```python
from build123d import *

# Parameters (mm, degrees)
BOSS_EXTRUDE1_DEPTH = 5.9944
CHAMFER1_SIZE       = 3.175


with BuildPart() as part:
    # Sketch1 → Boss-Extrude1 (new body)
    with BuildSketch(Plane(origin=(0, 0, 0), x_dir=(1, 0, 0), z_dir=(0, 1, 0))):
        Polygon((-53.975, 0), (-6.35, 0), (-6.35, -3.175), (-3.175, -3.175), (-3.175, 0), (0, 0), (0, 12.7), (-3.175, 12.7), (-3.175, 15.875), (-6.35, 15.875), (-6.35, 12.7), (-53.975, 12.7), (-53.975, 15.875), (-57.15, 15.875), (-57.15, 19.05), (-69.85, 19.05), (-69.85, 15.875), (-73.025, 15.875), (-73.025, 12.7), (-120.65, 12.7), (-120.65, 15.875), (-123.825, 15.875), (-123.825, 12.7), (-127, 12.7), (-127, 0), (-123.825, 0), (-123.825, -3.175), (-120.65, -3.175), (-120.65, 0), (-73.025, 0), (-73.025, -3.175), (-69.85, -3.175), (-69.85, -6.35), (-57.15, -6.35), (-57.15, -3.175), (-53.975, -3.175), align=None)
    extrude(amount=BOSS_EXTRUDE1_DEPTH)

    # Chamfer1
    chamfer1_edges = [part.edges().sort_by_distance(p)[0] for p in [
        (-6.35, 2.9972, -12.7),
        (-6.35, 2.9972, 0),
        (-120.65, 2.9972, 0),
        (-120.65, 2.9972, -12.7),
    ]]
    chamfer(chamfer1_edges, length=CHAMFER1_SIZE - 0.0001)  # a hair under: the kernel refuses the full size


solid = part.part
```
Read the model definition and answer for the solid it produces. Units are mm, in the model's axes. A direction names the side the tool comes from. Give positions to 0.01 mm unless a question says otherwise; leave off trailing zeros. Order: outer loops, then holes, each group sorted by start corner. A loop starts at its lowest first (then second) coordinate and runs counter-clockwise, first axis right, second up.
(1) For a pull along X with two mould halves and no side action, classify faces 4 (the flat face through (-96, 3, 0)), 5 (the flat face through (-56, 3, 3.175)), 6 (the flat face through (-123.825, 3, -14)), 7 (the flat face through (-3.175, 3, 2)) as released by +X, released by -X, zero draft, split by the parting line, or undercut.
(2) Given pin 1 (3 mm diameter, centred on x = -30, y = 2.5, fed in from +Z); pin 2 (2.5 mm diameter, centred on y = 2, z = 4, fed in from -X) (3 decimals); pin 3 (3 mm diameter, centred on x = -23.5, y = 2, fed in from -Z); pin 4 (10 mm diameter, centred on x = -44.5, z = -3.5, fed in from -Y), each flat-ended and moving along its own axis, determine where each tip first touches the part or whether it passes through.
(3) Straight lines are drawn through the part: L1, parallel to X at y = 3.3, z = 1 (3 decimals); L2, parallel to X at y = 5.3, z = 4.5; L3, parallel to Z at x = -10.5, y = 0.35. For each, find the intervals that lie inside material, in ascending order.
(4) Find section B-B (x = -39). Give the vertices of the cut face in (y, z).
(5) Find section A-A (z = 1.5). Give the vertices of the cut face in (x, y) (3 decimals), plus the area to 3 significant figures.
(6) For faces 1 (the flat face through (-2, 3, -12.7)), 2 (the flat face through (-69.85, 3, 5)), 3 (the flat face through (-119.04, 2.955, 1.565)), determine the directions among +Z, -Z, +X, -X, +Y, -Y from which every point of the face is accessible in a straight line to the end or side of a thin tool.
Result sheet:
1. face 4: undercut
1. face 5: zero draft
1. face 6: released by -X
1. face 7: released by +X
2. pin 1: stops at z = 0
2. pin 2: stops at x = -123.825
2. pin 3: stops at z = -12.7
2. pin 4: stops at y = 0
3. L1: x = -123.825 to -118.475, -73.025 to -53.975, -8.525 to -3.175
3. L2: x = -69.85 to -57.15
3. L3: z = -12.7 to 0
4. outline: (0, -12.7) - (5.99, -12.7) - (5.99, 0) - (0, 0) - close
5. outline: (-123.825, 0) - (-118.975, 0) - (-118.975, 5.994) - (-123.825, 5.994) - close; (-73.025, 0) - (-53.975, 0) - (-53.975, 5.994) - (-73.025, 5.994) - close; (-8.025, 0) - (-3.175, 0) - (-3.175, 5.994) - (-8.025, 5.994) - close
5. area: 172 mm2
6. face 1: -Z, +X, +Y, -Y
6. face 2: +Z, -X, +Y, -Y
6. face 3: +Z, +Y, -Y
